The model under review builds one solid part; all positions refer to its coordinate system, in mm. Face numbers are marked on the shaded views. A direction names the side the tool comes from. Coordinates: 2 decimals unless noted, no trailing zeros. Loops run counter-clockwise (first coordinate to the right, second up) from the corner with the lowest first, then second, coordinate; pieces in that order, holes last. Notation, with made-up numbers: (7, -8.5) - (47, -8.5) arc R12 ccw to (47, 5.5) - close; hole circle Ø4 at (12.5, -18.75). An arc over 180 degrees is marked (long way). Answer in a Markdown table with one row per item. Add a question column.
(1) For P1, Ø1.5, axis at x = 22, z = -13, coming from the +Y side; P2, Ø1.5, axis at x = 16.5, y = -18, coming from the -Z side; P3, Ø2.5, axis at x = -40.5, y = 0, coming from the -Z side, all flat-tipped, find the tip position at first contact; note any pin that passes through.
(2) We need section B-B on y = -14.5. Write out the cut boundary in (x, z), plus the area to 3 significant figures.
(3) We need section C-C on x = 34.5. Write out the cut boundary in (y, z).
(4) We need section D-D on z = -32.5. Write out the cut boundary in (x, y).
(5) For line 1 along X through (y, z) = (0, 35); line 2 along Z through (x, y) = (-9.5, 0.5); line 3 along Z through (x, y) = (-2, 17.5), list the stretches that pass through material, from the lowest coordinate up.
(6) We need section A-A on z = 0. Write out the cut boundary in (x, y).
(7) Machinability: for the marked faces 4 and 5, which of the approach directions +Z, -Z, +X, -X, +Y, -Y give a long, thin tool a straight path to every point of the face, cutting with its end or side? Answer none if there is none.
(8) Mouldability with a two-part tool opening along Z and no side actions: class the marked faces 1, 2 and 3 as +Z half, -Z half, draft (parallel to the pull), parting line (faces both ways), or undercut.
Autodesk Inventor part; units mm, degrees
ref_plane "Work Plane1" through (-38.5, 0, 40) normal (0, 0, 1) x (1, 0, 0)
ref_plane "YZ Plane" through (0, 0, 0) normal (1, 0, 0) x (0, 1, 0)
ref_plane "XZ Plane" through (0, 0, 0) normal (0, 1, 0) x (-1, 0, 0)
sketch "Sketch1" plane through (0, 0, 0) normal (0, 0, 1) x (1, 0, 0)
  line L0 (-44.5, 40) -> (-32.5, 40)
  line L1 (-32.5, 40) -> (-32.5, 22)
  line L2 (-32.5, 22) -> (44.5, 22)
  line L3 (44.5, 22) -> (44.5, 20)
  line L4 (44.5, 20) -> (-44.5, 20)
  line L5 (-44.5, 20) -> (-44.5, 40)
  line L6 (-62.3, 0) -> (62.3, 0)
  point P0 (0, 0)
  point P1 (0, 20)
  dimension "d0" = 12
  dimension "d1" = 89
  dimension "d2" = 40
  dimension "d3" = 44
  dimension "d4" = 80
revolve "Revolution1" add sketch "Sketch1" angle 360 about axis through (-10, 0, 0) along (1, 0, 0)
ref_plane "Work Plane1" through (-38.5, 0, 40) normal (0, 0, 1) x (1, 0, 0)
sketch "Sketch2" plane through (-38.5, 0, 40) normal (0, 0, 1) x (1, 0, 0)
  line L0 (-2, 0) -> (2, 0) construction
  line L1 (-6, -40) -> (-6, 40)
  line L2 (6, -40) -> (6, 40)
  line L3 (-6, 0) -> (6, 0) construction
  point P0 (38.5, 0)
  point P1 (0, 0)
  dimension "d6" = 4
hole "Hole1" at (-40.5, 0, 40) at (-36.5, 0, 40) direction (0, 0, -1) diameter 1.567 depth 8 tip angle 118
pattern_circular "Circular Pattern1" count 3 over 360 about axis through (0, 0, 0) along (1, 0, 0) of "Hole1"
properties part number "ALPHA_001157_EndNosePiece"
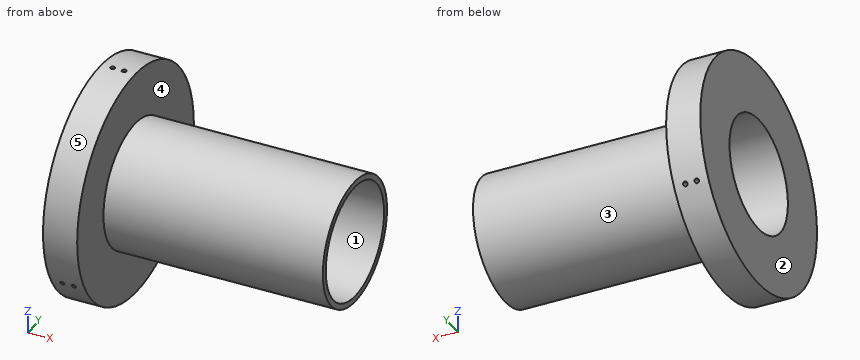
Outcome:
| question | item | result |
|---|---|---|
| 1 | P1 | y = 18.27 |
| 1 | P2 | z = -13.65 |
| 1 | P3 | z = -40 |
| 2 | outline | (-44.5, -37.28) - (-32.5, -37.28) - (-32.5, -16.55) - (44.5, -16.55) - (44.5, -13.77) - (-44.5, -13.77) - close; (-44.5, 13.77) - (44.5, 13.77) - (44.5, 16.55) - (-32.5, 16.55) - (-32.5, 37.28) - (-44.5, 37.28) - close |
| 2 | area | 991 mm² |
| 3 | outline | circle Ø44 at (0, 0); hole circle Ø40 at (0, 0) |
| 4 | outline | (-44.5, -23.32) - (-32.5, -23.32) - (-32.5, 23.32) - (-44.5, 23.32) - close |
| 5 | line 1 | -44.5 to -41.28, -39.72 to -37.28, -35.72 to -32.5 |
| 5 | line 2 | -21.99 to -19.99, 19.99 to 21.99 |
| 5 | line 3 | -13.33 to -9.68, 9.68 to 13.33 |
| 6 | outline | (-44.5, -40) - (-32.5, -40) - (-32.5, -22) - (44.5, -22) - (44.5, -20) - (-44.5, -20) - close; (-44.5, 20) - (44.5, 20) - (44.5, 22) - (-32.5, 22) - (-32.5, 40) - (-44.5, 40) - close |
| 7 | face 4 | +X |
| 7 | face 5 | +X, -X |
| 8 | face 1 | undercut |
| 8 | face 2 | draft |
| 8 | face 3 | parting line |
